Verification items for the finished model (mm, model axes). Face numbers are marked on the shaded views. Give positions to 0.01 mm unless a question says otherwise; leave off trailing zeros. Order: outer loops, then holes, each group sorted by start corner. A loop starts at its lowest first (then second) coordinate and runs counter-clockwise, first axis right, second up.
from build123d import *

# Parameters (mm, degrees)
SKETCH_W   = 125
SKETCH_H   = 119
SKETCH_R   = 8
SKETCH_R_2 = 3
PAD_DEPTH  = 10
FILLET_R   = 20


with BuildPart() as part:
    # Sketch → Pad (new body)
    with BuildSketch(Plane.XY):
        with Locations((-9.5, 100)):
            Rectangle(SKETCH_W, SKETCH_H)
        with Locations((-32, 100)):
            Circle(SKETCH_R, mode=Mode.SUBTRACT)
        with Locations((-57, 133)):
            Circle(SKETCH_R_2, mode=Mode.SUBTRACT)
        with Locations((-57, 67)):
            Circle(SKETCH_R_2, mode=Mode.SUBTRACT)
        with Locations((38, 133)):
            Circle(SKETCH_R_2, mode=Mode.SUBTRACT)
        with Locations((38, 67)):
            Circle(SKETCH_R_2, mode=Mode.SUBTRACT)
        with BuildLine():
            ThreePointArc((-4.5, 152.5), (-7.5, 149.5), (-4.5, 146.5))
            Line((-4.5, 146.5), (30.5, 146.5))
            ThreePointArc((30.5, 146.5), (33.5, 149.5), (30.5, 152.5))
            Line((-4.5, 152.5), (30.5, 152.5))
        make_face(mode=Mode.SUBTRACT)
        with BuildLine():
            ThreePointArc((-4.5, 119.5), (-7.5, 116.5), (-4.5, 113.5))
            Line((-4.5, 113.5), (30.5, 113.5))
            ThreePointArc((30.5, 113.5), (33.5, 116.5), (30.5, 119.5))
            Line((-4.5, 119.5), (30.5, 119.5))
        make_face(mode=Mode.SUBTRACT)
        with BuildLine():
            ThreePointArc((-4.5, 86.5), (-7.5, 83.5), (-4.5, 80.5))
            Line((-4.5, 80.5), (30.5, 80.5))
            ThreePointArc((30.5, 80.5), (33.5, 83.5), (30.5, 86.5))
            Line((-4.5, 86.5), (30.5, 86.5))
        make_face(mode=Mode.SUBTRACT)
        with BuildLine():
            ThreePointArc((-4.5, 53.5), (-7.5, 50.5), (-4.5, 47.5))
            Line((-4.5, 47.5), (30.5, 47.5))
            ThreePointArc((30.5, 47.5), (33.5, 50.5), (30.5, 53.5))
            Line((-4.5, 53.5), (30.5, 53.5))
        make_face(mode=Mode.SUBTRACT)
    extrude(amount=PAD_DEPTH)

    # Fillet
    fillet_edges = [part.edges().sort_by_distance(p)[0] for p in [
        (53, 40.5, 5),
        (53, 159.5, 5),
        (-72, 40.5, 5),
        (-72, 159.5, 5),
    ]]
    fillet(fillet_edges, radius=FILLET_R)


solid = part.part
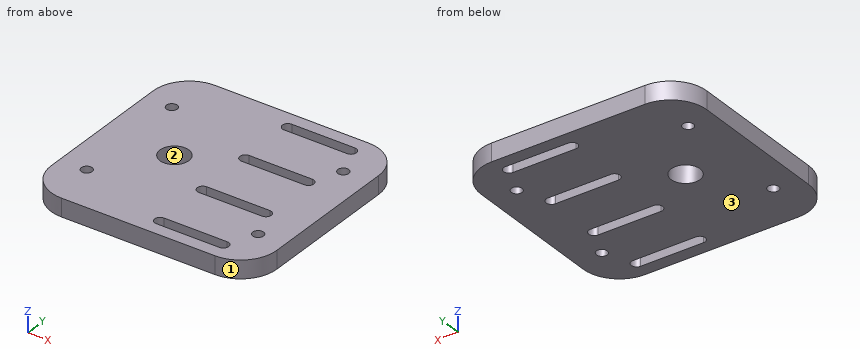
(1) Section check D-D, the plane z = 2.5. Give the number of separate pieces and of enclosed holes in the cut face, then the cut area to 3 significant figures.
Solved:
separate pieces: 1
enclosed holes: 9
area: 13,300 mm2
(2) Scan lines: line 1 (Y direction, x = 24, z = 8.25); line 2 (X direction, y = 133, z = 5.5); line 3 (Y direction, x = -32, z = 4). Record each from-to range of solid material in increasing order.
Solved:
line 1: y = 40.5 to 47.5, 53.5 to 80.5, 86.5 to 113.5, 119.5 to 146.5, 152.5 to 159.5
line 2: x = -72 to -60, -54 to 35, 41 to 53
line 3: y = 40.5 to 92, 108 to 159.5
(3) Go/stop test with a flat-tipped pin: pin 1 (1 mm diameter, centred on y = 142, z = 8.5, fed in from +X). Record where the tip stops, or that it passes through.
Solved:
pin 1: stops at x = 52.9
(4) Section check A-A, the plane x = 14. Enter the section's corners in (y, z).
Solved:
outline: (40.5, 0) - (47.5, 0) - (47.5, 10) - (40.5, 10) - close; (53.5, 0) - (80.5, 0) - (80.5, 10) - (53.5, 10) - close; (86.5, 0) - (113.5, 0) - (113.5, 10) - (86.5, 10) - close; (119.5, 0) - (146.5, 0) - (146.5, 10) - (119.5, 10) - close; (152.5, 0) - (159.5, 0) - (159.5, 10) - (152.5, 10) - close
(5) Section check B-B, the plane y = 83.5. Enter the section's corners in (x, z).
Solved:
outline: (-72, 0) - (-7.5, 0) - (-7.5, 10) - (-72, 10) - close; (33.5, 0) - (53, 0) - (53, 10) - (33.5, 10) - close
(6) Release check for a two-part mould opening along Y. For the marked faces 1, 2 and 3 record: pulls with the +Y half, pulls with the -Y half, needs draft (parallel to the pull), parting line crosses it, or undercut.
Solved:
face 1: pulls with the -Y half
face 2: undercut
face 3: needs draft
(7) Section check C-C, the plane y = 133. Enter the section's corners in (x, z), then the cut area to 3 significant figures.
Solved:
outline: (-72, 0) - (-60, 0) - (-60, 10) - (-72, 10) - close; (-54, 0) - (35, 0) - (35, 10) - (-54, 10) - close; (41, 0) - (53, 0) - (53, 10) - (41, 10) - close
area: 1,130 mm2
